from build123d import *

# Parameters (mm, degrees)
SKETCH2_W = 236.327347182
SKETCH2_H = 100
SKETCH3_W = 236.327347182
SKETCH3_H = 100
SKETCH4_W = 100
SKETCH4_H = 32.970724778


with BuildPart() as body_1:
    # Sketch2 → Surface-Plane1: a flat surface bounded by the sketch
    with BuildSketch(Plane(origin=(-0.173966376, 2.487835086, 0), x_dir=(0.9975640502598243, 0.06975647374412548, 0), z_dir=(0.06975647374412547, -0.9975640502598242, 0)), mode=Mode.PRIVATE) as surface_plane1_1_region:
        with Locations((82.49909721, 0)):
            Rectangle(SKETCH2_W, SKETCH2_H)
    surface_plane1_1 = surface_plane1_1_region.sketch.faces()[0]
    # Sketch7 → Surface-Plane3: a flat surface bounded by the sketch
    with BuildSketch(Plane.XY.offset(50), mode=Mode.PRIVATE) as surface_plane3_2_region:
        Polygon((-35.751665642, 0), (200, 16.485362389), (200, -16.485362389), align=None)
    surface_plane3_2 = surface_plane3_2_region.sketch.faces()[0]
    # Sketch3 → Surface-Plane2: a flat surface bounded by the sketch
    with BuildSketch(Plane(origin=(-0.173966376, -2.487835086, 0), x_dir=(0.9975640502598243, -0.06975647374412548, 0), z_dir=(-0.06975647374412547, -0.9975640502598242, 0)), mode=Mode.PRIVATE) as surface_plane2_3_region:
        with Locations((82.49909721, 0)):
            Rectangle(SKETCH3_W, SKETCH3_H)
    surface_plane2_3 = surface_plane2_3_region.sketch.faces()[0]
    # Sketch4 → Surface-Plane4: a flat surface bounded by the sketch
    with BuildSketch(Plane(origin=(200, 0, 0), x_dir=(0, 0, -1), z_dir=(1, 0, 0)), mode=Mode.PRIVATE) as surface_plane4_4_region:
        Rectangle(SKETCH4_W, SKETCH4_H)
    surface_plane4_4 = surface_plane4_4_region.sketch.faces()[0]
    # Sketch5 → Surface-Plane5: a flat surface bounded by the sketch
    with BuildSketch(Plane.XY.offset(-50), mode=Mode.PRIVATE) as surface_plane5_5_region:
        Polygon((-35.751665642, 0), (200, 16.485362389), (200, -16.485362389), align=None)
    surface_plane5_5 = surface_plane5_5_region.sketch.faces()[0]
    # Surface-Knit1: the surfaces knitted into a closed skin and filled: a solid
    add(Solid(Shell(Face.sew_faces(surface_plane1_1.faces() + surface_plane3_2.faces() + surface_plane2_3.faces() + surface_plane4_4.faces() + surface_plane5_5.faces())[0])))


solid = body_1.part
Work out the finished part from the listing and answer in its coordinate system (mm). Round coordinates to 2 decimals unless told otherwise and drop trailing zeros. Write each loop counter-clockwise with the first axis right and the second up, starting at its lowest first coordinate (ties: lowest second). Pieces come first, ordered by that corner, then holes.
1) A cutting plane is placed at C-C (y = 6). Give the vertices of the cut face in (x, z).
2) Given pin 1 Ø1 at (x, z) = (119.5, -40) entering from -Y; pin 2 Ø8 at (x, z) = (128.5, 22) entering from -Y; pin 3 Ø3 at (x, z) = (83.5, 8.5) entering from +Y, each flat-ended and moving along its own axis, determine where each tip first touches the part or whether it passes through.
3) A cutting plane is placed at B-B (x = 32.5). Give the vertices of the cut face in (y, z).
4) Straight lines are drawn through the part: line 1 (Y direction, x = 189, z = 1); line 2 (Y direction, x = 18, z = -31.5). For each, find the intervals that lie inside material, in ascending order.
5) A cutting plane is placed at A-A (z = -8). Give the vertices of the cut face in (x, y), plus the area to 3 significant figures.
Completed:
1. outline: (50.05, -50) - (200, -50) - (200, 50) - (50.05, 50) - close
2. pin 1: stops at y = -10.89
2. pin 2: stops at y = -11.77
2. pin 3: stops at y = 8.44
3. outline: (-4.77, -50) - (4.77, -50) - (4.77, 50) - (-4.77, 50) - close
4. line 1: y = -15.72 to 15.72
4. line 2: y = -3.76 to 3.76
5. outline: (-35.75, 0) - (200, -16.49) - (200, 16.49) - close
5. area: 3,890 mm2
